Job drawing, mm, ordinate dimensions from the low corner. One solid piece. Round coordinates to 2 decimals unless told otherwise and drop trailing zeros. Loops run counter-clockwise (first coordinate to the right, second up) from the corner with the lowest first, then second, coordinate; pieces in that order, holes last.
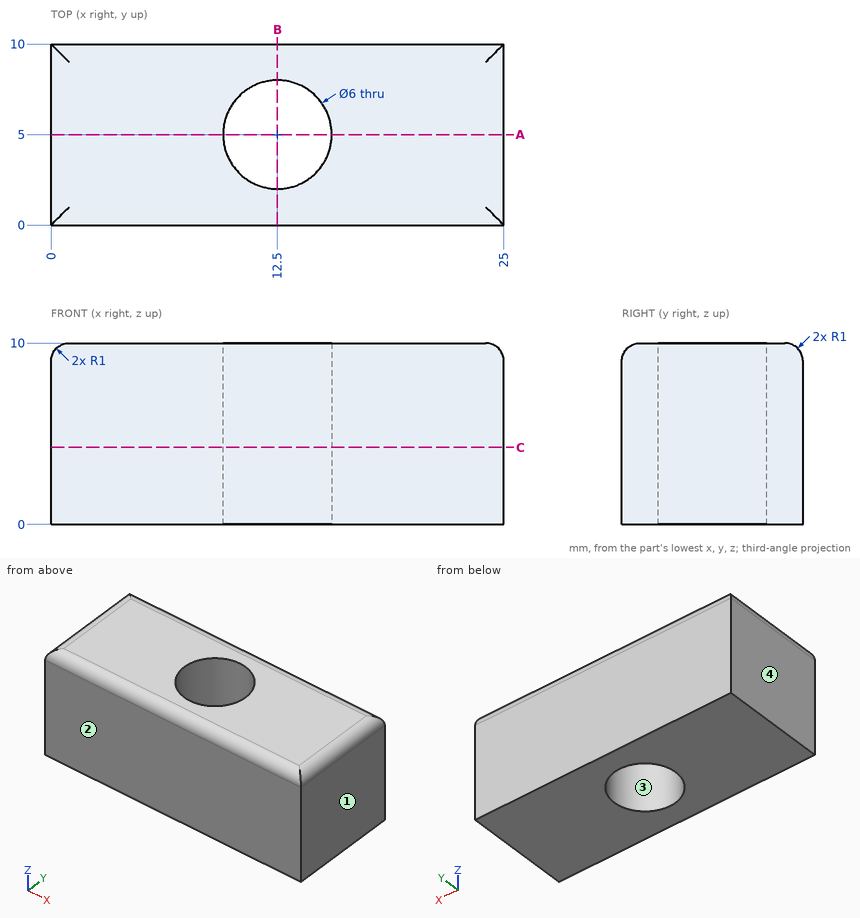
(1) Probe line 1 (Y direction, x = 12.5, z = 4.75); line 2 (X direction, y = 6.5, z = 4); line 3 (X direction, y = 5.5, z = 4.25). List the from-to ranges inside material, lowest first.
Responses:
line 1: y = 0 to 2, 8 to 10
line 2: x = 0 to 9.9, 15.1 to 25
line 3: x = 0 to 9.54, 15.46 to 25
(2) Slice it at C-C on z = 4.25. List the corners of the cut face in (x, y), plus the area to 3 significant figures.
Responses:
outline: (0, 0) - (25, 0) - (25, 10) - (0, 10) - close; hole circle Ø6 at (12.5, 5)
area: 222 mm2
(3) Slice it at A-A on y = 5. List the corners of the cut face in (x, z), plus the area to 3 significant figures.
Responses:
outline: (0, 0) - (9.5, 0) - (9.5, 10) - (1, 10) arc R1 ccw to (0, 9) - close; (15.5, 0) - (25, 0) - (25, 9) arc R1 ccw to (24, 10) - (15.5, 10) - close
area: 190 mm2
(4) Slice it at B-B on x = 12.5. List the corners of the cut face in (y, z), plus the area to 3 significant figures.
Responses:
outline: (0, 0) - (2, 0) - (2, 10) - (1, 10) arc R1 ccw to (0, 9) - close; (8, 0) - (10, 0) - (10, 9) arc R1 ccw to (9, 10) - (8, 10) - close
area: 39.6 mm2
(5) Pull direction X, two halves, no side cores. Call the marked faces 1, 2, 3 and 4: +X half, -X half, draft (parallel to the pull), parting line (faces both ways), or undercut.
Responses:
face 1: +X half
face 2: draft
face 3: undercut
face 4: -X half
